Design review of the part built by this model. Coordinates are the model's own, in mm. A direction names the side the tool comes from. Give positions to 0.01 mm unless a question says otherwise; leave off trailing zeros. Write each loop counter-clockwise with the first axis right and the second up, starting at its lowest first coordinate (ties: lowest second). Pieces come first, ordered by that corner, then holes. Notation, with made-up numbers: M -9.75,53 L 29.25,53 A14 ccw 29.25,58 Z; hole C -18.5,61 d6. An arc over 180 degrees is marked long. Use a Markdown table: item, result. Add a question column.
```python
from build123d import *

# Parameters (mm, degrees)
CROQUIS1_W              = 30
CROQUIS1_H              = 30
SALIENTE_EXTRUIR1_DEPTH = 200
CROQUIS2_R              = 2
CORTAR_EXTRUIR1_DEPTH   = 25
CROQUIS4_R              = 2
CORTAR_EXTRUIR3_DEPTH   = 25
CROQUIS5_W              = 10
CROQUIS5_H              = 8
CROQUIS5_W_2            = 8
CROQUIS5_H_2            = 10
CORTAR_EXTRUIR4_DEPTH   = 200


with BuildPart() as part:
    # Croquis1 → Saliente-Extruir1 (new body)
    with BuildSketch(Plane.XY):
        Rectangle(CROQUIS1_W, CROQUIS1_H)
    extrude(amount=SALIENTE_EXTRUIR1_DEPTH)

    # Croquis2 → Cortar-Extruir1 (cut)
    with BuildSketch(Plane.XY.offset(200)):
        with Locations((-7.221825407, 7.221825407)):
            Circle(CROQUIS2_R)
        with Locations(Location((7.221825407, -7.221825407, 0), (0, 0, 180))):
            Circle(CROQUIS2_R)
    extrude(amount=-CORTAR_EXTRUIR1_DEPTH, mode=Mode.SUBTRACT)

    # Croquis4 → Cortar-Extruir3 (cut)
    with BuildSketch(Plane(origin=(0, 0, 0), x_dir=(-1, 0, 0), z_dir=(0, 0, -1))):
        Circle(CROQUIS4_R)
    extrude(amount=-CORTAR_EXTRUIR3_DEPTH, mode=Mode.SUBTRACT)

    # Croquis5 → Cortar-Extruir4 (cut)
    with BuildSketch(Plane(origin=(0, 0, 0), x_dir=(-1, 0, 0), z_dir=(0, 0, -1))):
        with Locations((0, -15)):
            Rectangle(CROQUIS5_W, CROQUIS5_H)
        with Locations((15, 0)):
            Rectangle(CROQUIS5_W_2, CROQUIS5_H_2)
    extrude(amount=-CORTAR_EXTRUIR4_DEPTH, mode=Mode.SUBTRACT)


solid = part.part
```
(1) Add section A-A on x = -13. Give the boundary of the cut face in (y, z).
(2) Add section C-C on z = 139.5. Give the boundary of the cut face in (x, y).
(3) Machinability: for faces 1 (the flat face through (0, -11, 99)), 2 (the flat face through (-13, -5, 99)), 3 (the flat face through (0, 0, 25)), 4 (the flat face through (10, -15, 99)), 5 (the flat face through (7, -7, 175)), which of the approach directions +Z, -Z, +X, -X, +Y, -Y give a long, thin tool a straight path to every point of the face, cutting with its end or side? Answer none if there is none.
(4) For pin 1 (8 mm diameter, centred on x = 0, z = 100, fed in from -Y); pin 2 (1.2 mm diameter, centred on x = -8, y = 7, fed in from +Z); pin 3 (8 mm diameter, centred on y = -0.5, z = 117, fed in from -X), all flat-tipped, find the tip position at first contact; note any pin that passes through.
(5) The part is to be moulded in two halves that separate along X. For faces 6 (the cylindrical face through (-8.7, 8.57, 187.68)), 7 (the flat face through (-11, 0, 99)), 8 (the flat face through (3, 0, 0)), 9 (the flat face through (5, -13, 99)), say which applies: released by +X, released by -X, zero draft, split by the parting line, or undercut.
(6) Add section B-B on y = 0. Give the boundary of the cut face in (x, z), then the cut area to 3 significant figures.
(7) Wall thickness on L1, parallel to Y at x = -11.75, z = 111; L2, parallel to Y at x = 0, z = 9.75; L3, parallel to Y at x = 3.5, z = 86: over which ranges is each line inside the solid? List them lowest first.
From the geometry:
| question | item | result |
|---|---|---|
| 1 | outline | M -15,0 L -5,0 L -5,200 L -15,200 Z; M 5,0 L 15,0 L 15,200 L 5,200 Z |
| 2 | outline | M -15,-15 L -5,-15 L -5,-11 L 5,-11 L 5,-15 L 15,-15 L 15,15 L -15,15 L -15,5 L -11,5 L -11,-5 L -15,-5 Z |
| 3 | face 1 | +Z, -Z, -Y |
| 3 | face 2 | +Z, -Z, -X |
| 3 | face 3 | -Z |
| 3 | face 4 | +Z, -Z, +X, -X, -Y |
| 3 | face 5 | +Z |
| 4 | pin 1 | stops at y = -11 |
| 4 | pin 2 | stops at z = 175 |
| 4 | pin 3 | stops at x = -11 |
| 5 | face 6 | undercut |
| 5 | face 7 | released by -X |
| 5 | face 8 | zero draft |
| 5 | face 9 | undercut |
| 6 | outline | M -11,0 L -2,0 L -2,25 L 2,25 L 2,0 L 15,0 L 15,200 L -11,200 Z |
| 6 | area | 5,100 mm^2 |
| 7 | L1 | y = -15 to -5, 5 to 15 |
| 7 | L2 | y = -11 to -2, 2 to 15 |
| 7 | L3 | y = -11 to 15 |
